Job drawing, mm, ordinate dimensions from the low corner. One solid piece. A direction names the side the tool comes from. Coordinates: 2 decimals unless noted, no trailing zeros. Order: outer loops, then holes, each group sorted by start corner. A loop starts at its lowest first (then second) coordinate and runs counter-clockwise, first axis right, second up. Notation, with made-up numbers: (36, 46.5) - (46, 46.5) arc R30 ccw to (46, 68.5) - close; hole circle Ø1 at (-29, 44). An arc over 180 degrees is marked (long way). Return JSON: item names as keys, results as strings.
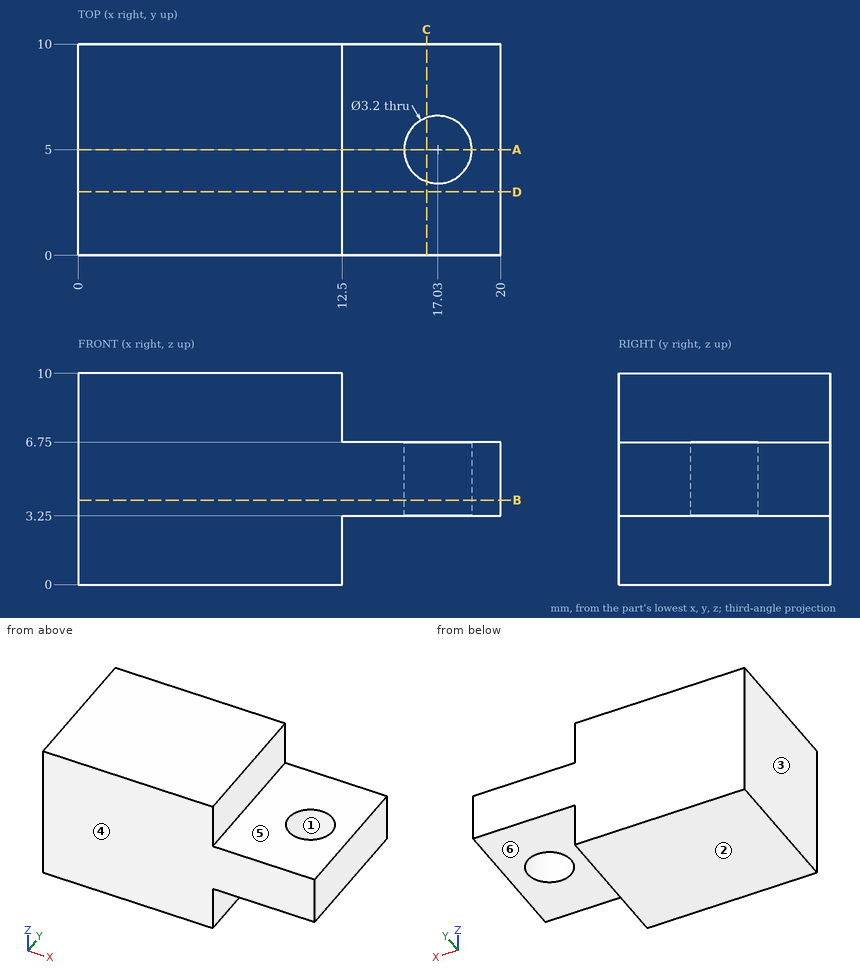
1. Cut at C-C on x = 16.5. Give the cut face in (y, z).
Check values:
{"outline": "(0, 3.25) - (3.49, 3.25) - (3.49, 6.75) - (0, 6.75) - close; (6.51, 3.25) - (10, 3.25) - (10, 6.75) - (6.51, 6.75) - close"}
2. Cut at B-B on z = 4. Give the cut face in (x, y).
Check values:
{"outline": "(0, 0) - (20, 0) - (20, 10) - (0, 10) - close; hole circle Ø3.2 at (17.03, 5)"}
3. Drop flat-ended pins along their axis: pin 1 (3.5 mm diameter, centred on x = 17.03, y = 5, fed in from +Z); pin 2 (2 mm diameter, centred on x = 17.5, y = 7, fed in from -Z); pin 3 (1.5 mm diameter, centred on y = 6.5, z = 5, fed in from -X); pin 4 (1.6 mm diameter, centred on y = 6, z = 9, fed in from +X). Give the stop position or say it passes through.
Check values:
{"pin 1": "z = 6.75", "pin 2": "z = 3.25", "pin 3": "x = 0", "pin 4": "x = 12.5"}
4. Cut at D-D on y = 3. Give the cut face in (x, z), plus the area to 3 significant figures.
Check values:
{"outline": "(0, 0) - (12.5, 0) - (12.5, 3.25) - (20, 3.25) - (20, 6.75) - (12.5, 6.75) - (12.5, 10) - (0, 10) - close", "area": "151 mm²"}
5. Mould opens along X. For the marked faces 1, 2 and 3 say: pulls with the +X half, pulls with the -X half, needs draft (parallel to the pull), parting line crosses it, or undercut.
Check values:
{"face 1": "undercut", "face 2": "needs draft", "face 3": "pulls with the -X half"}
6. Cut at A-A on y = 5. Give the cut face in (x, z).
Check values:
{"outline": "(0, 0) - (12.5, 0) - (12.5, 3.25) - (15.43, 3.25) - (15.43, 6.75) - (12.5, 6.75) - (12.5, 10) - (0, 10) - close; (18.63, 3.25) - (20, 3.25) - (20, 6.75) - (18.63, 6.75) - close"}
7. Probe L1, parallel to X at y = 4, z = 2.25; L2, parallel to Z at x = 15.25, y = 0.5. List the from-to ranges inside material, lowest first.
Check values:
{"L1": "0 to 12.5", "L2": "3.25 to 6.75"}
8. Tool access for the marked faces 4, 5 and 6: list every direction of +Z, -Z, +X, -X, +Y, -Y with a clear straight run to the whole face (end or side of a thin tool).
Check values:
{"face 4": "+Z, -Z, +X, -X, -Y", "face 5": "+Z, +X, +Y, -Y", "face 6": "-Z, +X, +Y, -Y"}
